Design review of the part shown in the three views and the two pictorial views. Dimensions are in mm from the part's minimum x, y and z. Round coordinates to 2 decimals unless told otherwise and drop trailing zeros. Order: outer loops, then holes, each group sorted by start corner. A loop starts at its lowest first (then second) coordinate and runs counter-clockwise, first axis right, second up. Notation, with made-up numbers: (-19, -2) - (10, -2) arc R15 ccw to (10, 16) - close; hole circle Ø1 at (33.5, 21). An arc over 180 degrees is marked (long way). Use CSV: the item, a comma, the result in double quotes.
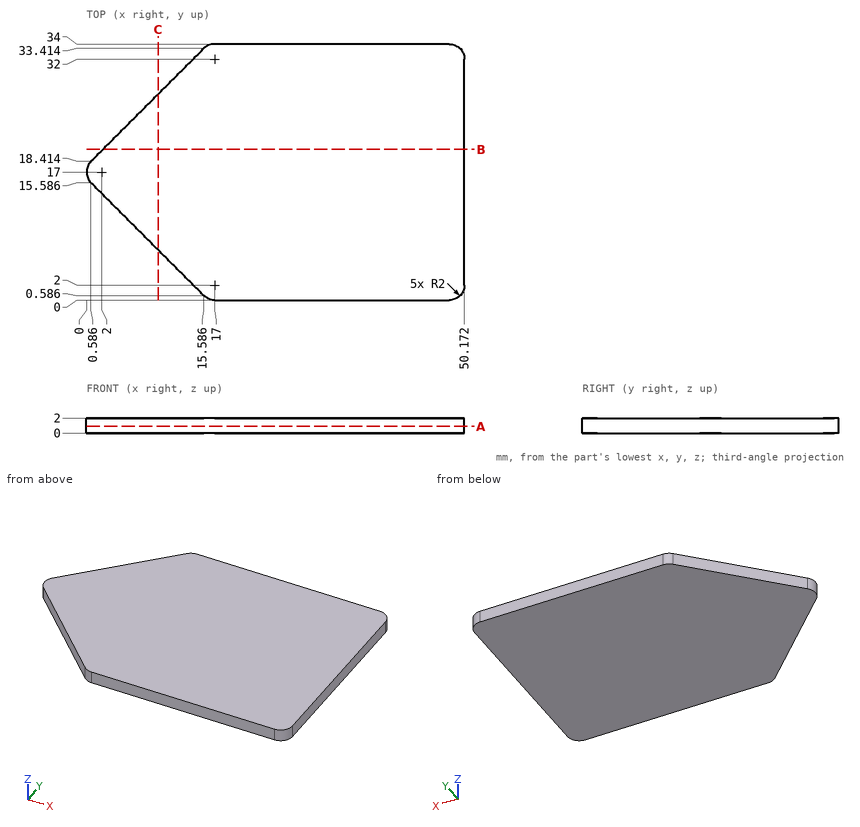
1) We need section B-B (y = 20). Give the boundary of the cut face in (x, z).
Data:
outline,"(2.17, 0) - (50.17, 0) - (50.17, 2) - (2.17, 2) - close"
2) We need section C-C (x = 9.5). Give the boundary of the cut face in (y, z).
Data:
outline,"(6.67, 0) - (27.33, 0) - (27.33, 2) - (6.67, 2) - close"
3) Insertion check: pin 1 Ø1 at (x, z) = (17, 1) entering from -Y. The pin has a flat end and moves straight along its axis. Give the tip position at first contact, or say it passes through.
Data:
pin 1,"stops at y = 0"
4) We need section A-A (z = 0.9). Give the boundary of the cut face in (x, y) (1 decimal), then the cut area to 3 significant figures.
Data:
outline,"(0.6, 15.6) - (15.6, 0.6) arc R2 ccw to (17, 0) - (48.2, 0) arc R2 ccw to (50.2, 2) - (50.2, 32) arc R2 ccw to (48.2, 34) - (17, 34) arc R2 ccw to (15.6, 33.4) - (0.6, 18.4) arc R2 ccw to start"
area,"1,440 mm2"
5) To check wall thickness, follow L1, parallel to X at y = 4.5, z = 1.05; L2, parallel to Y at x = 2, z = 1.6; L3, parallel to X at y = 7.5, z = 1.8. State the ranges of each line that lie inside material, in increasing order. Write a range as from..to.
Data:
L1,"x = 11.67..50.17"
L2,"y = 14.17..19.83"
L3,"x = 8.67..50.17"
